from build123d import *

# Parameters (mm, degrees)
CYLINDER003_R     = 1.7
CYLINDER003_DEPTH = 20
CYLINDER005_R     = 1.7
CYLINDER005_DEPTH = 20
CYLINDER002_R     = 1.7
CYLINDER002_DEPTH = 20
CYLINDER_R        = 13.7
CYLINDER_DEPTH    = 50
BOX_W             = 48
BOX_H             = 65
BOX_DEPTH         = 10


with BuildPart() as cylinder003:
    # Cylinder003 → Cylinder003 (new body)
    with BuildSketch(Plane(origin=(3.4, 59, -5), x_dir=(1, 0, 0), z_dir=(0, 0, 1))):
        Circle(CYLINDER003_R)
    extrude(amount=CYLINDER003_DEPTH)


with BuildPart() as cylinder005:
    # Cylinder005 → Cylinder005 (new body)
    with BuildSketch(Plane(origin=(3.4, 6, -5), x_dir=(1, 0, 0), z_dir=(0, 0, 1))):
        Circle(CYLINDER005_R)
    extrude(amount=CYLINDER005_DEPTH)


with BuildPart() as cylinder002:
    # Cylinder002 → Cylinder002 (new body)
    with BuildSketch(Plane(origin=(3.4, 32.5, -5), x_dir=(1, 0, 0), z_dir=(0, 0, 1))):
        Circle(CYLINDER002_R)
    extrude(amount=CYLINDER002_DEPTH)


with BuildPart() as cylinder:
    # Cylinder → Cylinder (new body)
    with BuildSketch(Plane(origin=(28, 32.5, -5), x_dir=(1, 0, 0), z_dir=(0, 0, 1))):
        Circle(CYLINDER_R)
    extrude(amount=CYLINDER_DEPTH)


with BuildPart() as cut003:
    # Box → Box (new body)
    with BuildSketch(Plane.XY):
        with Locations((24, 32.5)):
            Rectangle(BOX_W, BOX_H)
    extrude(amount=BOX_DEPTH)

    # Cut: cut Cylinder
    add(cylinder.part, mode=Mode.SUBTRACT)

    # Cut001: cut Cylinder002
    add(cylinder002.part, mode=Mode.SUBTRACT)

    # Cut002: cut Cylinder005
    add(cylinder005.part, mode=Mode.SUBTRACT)

    # Cut003: cut Cylinder003
    add(cylinder003.part, mode=Mode.SUBTRACT)


solid = cut003.part
Work out the finished part from the listing and answer in its coordinate system (mm). Give positions to 0.01 mm unless a question says otherwise; leave off trailing zeros. Loops run counter-clockwise (first coordinate to the right, second up) from the corner with the lowest first, then second, coordinate; pieces in that order, holes last. Notation, with made-up numbers: (46, 37) - (69, 37) arc R8 cw to (69, 45) - close; hole circle Ø6 at (-25, -18.5). An arc over 180 degrees is marked (long way). Answer in a Markdown table with one row per item. Add a question column.
Q1. The part is cut by section A-A (y = 32.5). Determine the outline of the cut face in (x, z).
Q2. The part is cut by section B-B (x = 28). Determine the outline of the cut face in (y, z).
Q3. Consider line 1 along X through (y, z) = (32.5, 7.5); line 2 along Y through (x, z) = (3.4, 6); line 3 along X through (y, z) = (59, 0.5). Determine where each line is inside the solid, lowest interval first.
Q4. The part is cut by section C-C (z = 7.75). Determine the outline of the cut face in (x, y).
Q5. The part is cut by section D-D (y = 59). Determine the outline of the cut face in (x, z), and give its area (3 significant figures).
Q6. Determine the mould class of faces 1 (the cylindrical face through (3.03, 4.34, 4.93)), 2 (the flat face through (48, 32, 5)), 3 (the flat face through (13, 33, 10)), 4 (the cylindrical face through (3.03, 30.84, 4.93)) for opening direction X: released by +X, released by -X, zero draft, split by the parting line, or undercut.
Solution:
| question | item | result |
|---|---|---|
| 1 | outline | (0, 0) - (1.7, 0) - (1.7, 10) - (0, 10) - close; (5.1, 0) - (14.3, 0) - (14.3, 10) - (5.1, 10) - close; (41.7, 0) - (48, 0) - (48, 10) - (41.7, 10) - close |
| 2 | outline | (0, 0) - (18.8, 0) - (18.8, 10) - (0, 10) - close; (46.2, 0) - (65, 0) - (65, 10) - (46.2, 10) - close |
| 3 | line 1 | x = 0 to 1.7, 5.1 to 14.3, 41.7 to 48 |
| 3 | line 2 | y = 0 to 4.3, 7.7 to 30.8, 34.2 to 57.3, 60.7 to 65 |
| 3 | line 3 | x = 0 to 1.7, 5.1 to 48 |
| 4 | outline | (0, 0) - (48, 0) - (48, 65) - (0, 65) - close; hole circle Ø3.4 at (3.4, 6); hole circle Ø3.4 at (3.4, 32.5); hole circle Ø3.4 at (3.4, 59); hole circle Ø27.4 at (28, 32.5) |
| 5 | outline | (0, 0) - (1.7, 0) - (1.7, 10) - (0, 10) - close; (5.1, 0) - (48, 0) - (48, 10) - (5.1, 10) - close |
| 5 | area | 446 mm² |
| 6 | face 1 | undercut |
| 6 | face 2 | released by +X |
| 6 | face 3 | zero draft |
| 6 | face 4 | undercut |
